The model under review builds one solid part; all positions refer to its coordinate system, in mm. A direction names the side the tool comes from. Round coordinates to 2 decimals unless told otherwise and drop trailing zeros. Loops run counter-clockwise (first coordinate to the right, second up) from the corner with the lowest first, then second, coordinate; pieces in that order, holes last. Notation, with made-up numbers: (76, 25) -> (81, 25) arc R14 cw to (81, 33) -> close; hole circle Ø6 at (-31.75, 57). An arc over 180 degrees is marked (long way). Write each question's results on one line, items separated by ' | '. Start each with the question number.
Item 1: For L1, parallel to X at y = -15.5, z = 2.75; L2, parallel to Y at x = -1, z = 2; L3, parallel to Y at x = 34.5, z = 4, list the stretches that pass through material, from the lowest coordinate up. Write a range as from..to.
Item 2: Clearance check with flat-ended pins moving along their axes: pin 1 Ø8 at (x, y) = (-21, 12) entering from -Z; pin 2 Ø5 at (x, z) = (-29, 6) entering from +Y; pin 3 Ø1 at (y, z) = (-12.5, 4.5) entering from -X; pin 4 Ø5 at (y, z) = (-17.5, 5.5) entering from +X. State where each tip first meets the part, or that it passes through.
Item 3: We need section C-C (x = 26.5). Give the boundary of the cut face in (y, z).
Item 4: Mouldability with a two-part tool opening along X and no side actions: class faces 4 (the flat face through (-40, -24, 5)), 5 (the flat face through (27, -25, 5)), 6 (the flat face through (17, 6, 5)), 7 (the flat face through (-1, 2.5, 5)) as pulls with the +X half, pulls with the -X half, needs draft (parallel to the pull), parting line crosses it, or undercut.
Item 5: Tool access review of faces 1 (the flat face through (14.5, 16, 5)), 2 (the flat face through (-15.5, -15, 5)), 3 (the flat face through (-32, -22.5, 5)): name each direction out of +Z, -Z, +X, -X, +Y, -Y from which nothing blocks a thin tool from reaching the whole face with its end or side.
Item 6: We need section A-A (y = -9). Give the boundary of the cut face in (x, z), and give its area (3 significant figures).
Item 7: We need section B-B (z = 5.75). Give the boundary of the cut face in (x, y).
from build123d import *

# Parameters (mm, degrees)
F0_W     = 22
F0_H     = 2.5
F0_W_2   = 30
F0_W_3   = 23
F0_W_4   = 2.5
F1_DEPTH = 10
F2_R     = 5


with BuildPart() as f1:
    # F0 (on Top) → F1 (new body)
    with BuildSketch(Plane.XY):
        Polygon((-15.5, 2.5), (-15.5, 30), (-18, 30), (-18, -22.5), (-15.5, -22.5), (-15.5, 0), align=None)
        with Locations((-29, -23.75)):
            Rectangle(F0_W, F0_H)
        with Locations((-0.5, 1.25)):
            Rectangle(F0_W_2, F0_H)
        Polygon((14.5, 30), (14.5, 2.5), (14.5, 0), (14.5, -22.5), (17, -22.5), (17, 30), align=None)
        with Locations((28.5, -23.75)):
            Rectangle(F0_W_3, F0_H)
        with Locations((15.75, -23.75)):
            Rectangle(F0_W_4, F0_H)
        with Locations((-16.75, -23.75)):
            Rectangle(F0_W_4, F0_H)
    extrude(amount=F1_DEPTH)

    # F2
    f2_edges = [f1.edges().sort_by_distance(p)[0] for p in [
        (-18, -22.5, 5),
        (17, -22.5, 5),
        (14.5, 0, 5),
        (-15.5, 0, 5),
    ]]
    fillet(f2_edges, radius=F2_R)


solid = f1.part
Here are the results:
1) L1: x = -18..-15.5, 14.5..17 | L2: y = 0..2.5 | L3: y = -25..-22.5
2) pin 1: stops at z = 0 | pin 2: stops at y = -22.5 | pin 3: stops at x = -18 | pin 4: stops at x = 17.67
3) outline: (-25, 0) -> (-22.5, 0) -> (-22.5, 10) -> (-25, 10) -> close
4) face 4: pulls with the -X half | face 5: needs draft | face 6: pulls with the +X half | face 7: undercut
5) face 1: +Z, -Z, +Y | face 2: +Z, -Z, -Y | face 3: +Z, -Z, -X, +Y
6) outline: (-18, 0) -> (-15.5, 0) -> (-15.5, 10) -> (-18, 10) -> close; (14.5, 0) -> (17, 0) -> (17, 10) -> (14.5, 10) -> close | area: 50.0 mm2
7) outline: (-40, -25) -> (-15.5, -25) -> (-15.5, -5) arc R5 cw to (-10.5, 0) -> (9.5, 0) arc R5 cw to (14.5, -5) -> (14.5, -25) -> (40, -25) -> (40, -22.5) -> (22, -22.5) arc R5 cw to (17, -17.5) -> (17, 30) -> (14.5, 30) -> (14.5, 2.5) -> (-15.5, 2.5) -> (-15.5, 30) -> (-18, 30) -> (-18, -17.5) arc R5 cw to (-23, -22.5) -> (-40, -22.5) -> close
